from build123d import *

# Parameters (mm, degrees)
F2_R = 0.5
F3_R = 0.5
F4_R = 0.5


with BuildPart() as f1:
    # F0 (on Front) → F1 (revolve)
    with BuildSketch(Plane.XZ):
        Polygon((-50, 0), (0, 0), (0, 3), (-48, 3), (-48, 6), (-50, 6), align=None)
    revolve(axis=Axis((0, 0, 1.5), (0, 0, -1)))

    # F2
    f2_edges = [f1.edges().sort_by_distance(p)[0] for p in [
        (50, 0, 6),
    ]]
    fillet(f2_edges, radius=F2_R)

    # F3
    f3_edges = [f1.edges().sort_by_distance(p)[0] for p in [
        (48, 0, 6),
    ]]
    fillet(f3_edges, radius=F3_R)

    # F4
    f4_edges = [f1.edges().sort_by_distance(p)[0] for p in [
        (48, 0, 3),
    ]]
    fillet(f4_edges, radius=F4_R)


solid = f1.part
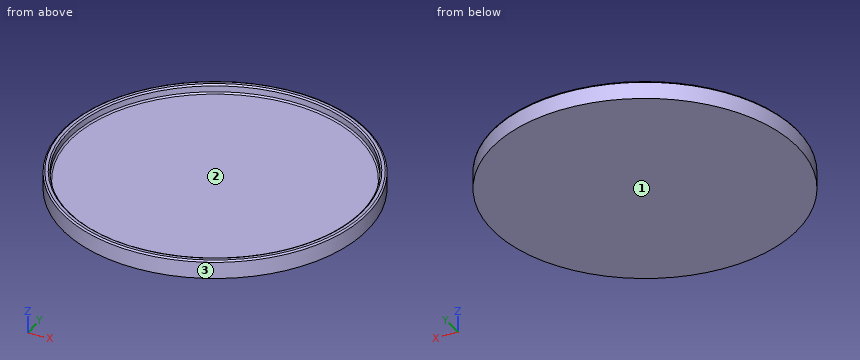
Design review of the part built by this model. Coordinates are the model's own, in mm. Face numbers are marked on the shaded views. Give positions to 0.01 mm unless a question says otherwise; leave off trailing zeros. Write each loop counter-clockwise with the first axis right and the second up, starting at its lowest first coordinate (ties: lowest second). Pieces come first, ordered by that corner, then holes. Notation, with made-up numbers: M 58,-40 L 102,-40 A20 ccw 102,-27 Z; hole C 0.5,79 d2. An arc over 180 degrees is marked long. Return JSON: item names as keys, results as strings. Group by question number.
Item 1: The part is to be moulded in two halves that separate along Y. For the marked faces 1, 2 and 3, say which applies: pulls with the +Y half, pulls with the -Y half, needs draft (parallel to the pull), parting line crosses it, or undercut.
Item 2: Take a section at B-B (z = 4.4). Give the boundary of the cut face in (x, y).
Item 3: Clearance check with flat-ended pins moving along their axes: pin 1 Ø6 at (x, y) = (-28.5, 21) entering from +Z; pin 2 Ø2 at (y, z) = (-21.5, 4.5) entering from -X; pin 3 Ø3 at (y, z) = (-40, 5) entering from -X. State where each tip first meets the part, or that it passes through.
Item 4: Wall thickness on line 1 along Y through (x, z) = (0, 4.2); line 2 along Z through (x, y) = (43.5, -15); line 3 along Y through (x, z) = (43, 5.6): over which ranges is each line inside the solid? List them lowest first.
Item 5: Take a section at A-A (x = 0). Give the boundary of the cut face in (y, z), plus the area to 3 significant figures.
Return value:
{
 "1": {"face 1": "needs draft", "face 2": "undercut", "face 3": "parting line crosses it"},
 "2": {"outline": "C 0,0 d100; hole C 0,0 d96"},
 "3": {"pin 1": "stops at z = 3", "pin 2": "stops at x = -45.6", "pin 3": "stops at x = -31.9"},
 "4": {"line 1": "y = -50 to -48, 48 to 50", "line 2": "z = 0 to 3", "line 3": "y = -25.49 to -21.35, 21.35 to 25.49"},
 "5": {"outline": "M -50,0 L 50,0 L 50,5.5 A0.5 ccw 49.5,6 L 48.5,6 A0.5 ccw 48,5.5 L 48,3.5 A0.5 cw 47.5,3 L -47.5,3 A0.5 cw -48,3.5 L -48,5.5 A0.5 ccw -48.5,6 L -49.5,6 A0.5 ccw -50,5.5 Z", "area": "312 mm2"}
}
